from build123d import *

# Parameters (mm, degrees)
F0_W     = 101.725624
F0_H     = 79.91349
F1_DEPTH = 28.448
F2_R     = 28.687359
F3_DEPTH = 57.658
F4_R     = 22.607538
F5_DEPTH = 70.866


with BuildPart() as f1:
    # F0 (on Front) → F1 (new body)
    with BuildSketch(Plane.XZ):
        Rectangle(F0_W, F0_H)
    extrude(amount=F1_DEPTH)

    # F2 (on Front) → F3 (join)
    with BuildSketch(Plane.XZ):
        Circle(F2_R)
    extrude(amount=F3_DEPTH)

    # F4 (on Front) → F5 (cut)
    with BuildSketch(Plane.XZ):
        Circle(F4_R)
    extrude(amount=F5_DEPTH, mode=Mode.SUBTRACT)


solid = f1.part
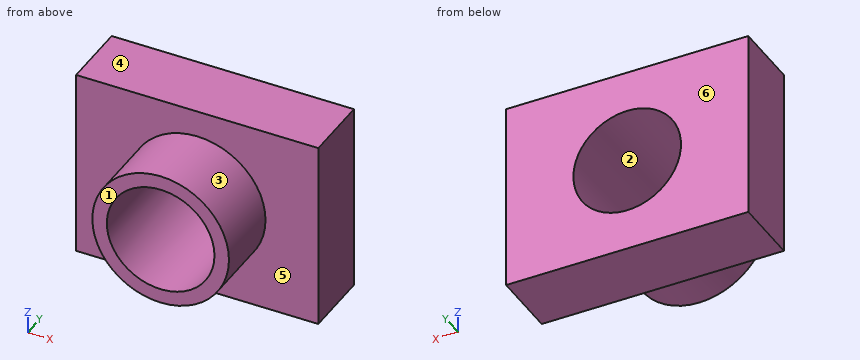
For this review, take the finished solid that the model builds, in its own axes (mm). Face numbers are marked on the shaded views. A direction names the side the tool comes from. Coordinates: 2 decimals unless noted, no trailing zeros. Loops run counter-clockwise (first coordinate to the right, second up) from the corner with the lowest first, then second, coordinate; pieces in that order, holes last. Notation, with made-up numbers: (81, 15) - (95, 15) arc R17 ccw to (95, 21) - close; hole circle Ø10 at (-6, 12.5). An arc over 180 degrees is marked (long way). Return JSON: item names as keys, results as strings.
Item 1: Take a section at C-C (y = -45). Give the boundary of the cut face in (x, z), then the cut area to 3 significant figures.
Determined:
{"outline": "circle Ø57.37 at (0, 0); hole circle Ø45.22 at (0, 0)", "area": "980 mm2"}
Item 2: Insertion check: pin 1 (1 mm diameter, centred on y = -43.5, z = 22.5, fed in from -X); pin 2 (1 mm diameter, centred on y = -45, z = -11.5, fed in from -X); pin 3 (6 mm diameter, centred on y = -50.5, z = -4.5, fed in from +X). Each pin has a flat end and moves straight along its axis. Give the tip position at first contact, or say it passes through.
Determined:
{"pin 1": "stops at x = -18.41", "pin 2": "stops at x = -26.49", "pin 3": "stops at x = 28.65"}
Item 3: Take a section at B-B (z = 0). Give the boundary of the cut face in (x, y), then the cut area to 3 significant figures.
Determined:
{"outline": "(-50.86, -28.45) - (-28.69, -28.45) - (-28.69, -57.66) - (-22.61, -57.66) - (-22.61, 0) - (-50.86, 0) - close; (22.61, -57.66) - (28.69, -57.66) - (28.69, -28.45) - (50.86, -28.45) - (50.86, 0) - (22.61, 0) - close", "area": "1,960 mm2"}
Item 4: For the marked faces 5 and 6, list the 3-axis set-ups (+Z, -Z, +X, -X, +Y, -Y) from which the entire face can be reached by the end or side of a thin tool; tool diameter is ignored.
Determined:
{"face 5": "-Y", "face 6": "+Z, -Z, +X, -X, +Y"}
Item 5: Take a section at D-D (x = 41). Give the boundary of the cut face in (y, z), then the cut area to 3 significant figures.
Determined:
{"outline": "(-28.45, -39.96) - (0, -39.96) - (0, 39.96) - (-28.45, 39.96) - close", "area": "2,270 mm2"}
Item 6: Take a section at A-A (x = 0). Give the boundary of the cut face in (y, z), then the cut area to 3 significant figures.
Determined:
{"outline": "(-57.66, -28.69) - (-28.45, -28.69) - (-28.45, -39.96) - (0, -39.96) - (0, -22.61) - (-57.66, -22.61) - close; (-57.66, 22.61) - (0, 22.61) - (0, 39.96) - (-28.45, 39.96) - (-28.45, 28.69) - (-57.66, 28.69) - close", "area": "1,340 mm2"}
Item 7: For line 1 (X direction, y = -24.5, z = 0); line 2 (Z direction, x = 0, y = -29.5), list the stretches that pass through material, from the lowest coordinate up.
Determined:
{"line 1": "x = -50.86 to -22.61, 22.61 to 50.86", "line 2": "z = -28.69 to -22.61, 22.61 to 28.69"}
Item 8: Mouldability with a two-part tool opening along Z and no side actions: class the marked faces 1, 2, 3 and 4 as pulls with the +Z half, pulls with the -Z half, needs draft (parallel to the pull), parting line crosses it, or undercut.
Determined:
{"face 1": "needs draft", "face 2": "undercut", "face 3": "parting line crosses it", "face 4": "pulls with the +Z half"}
